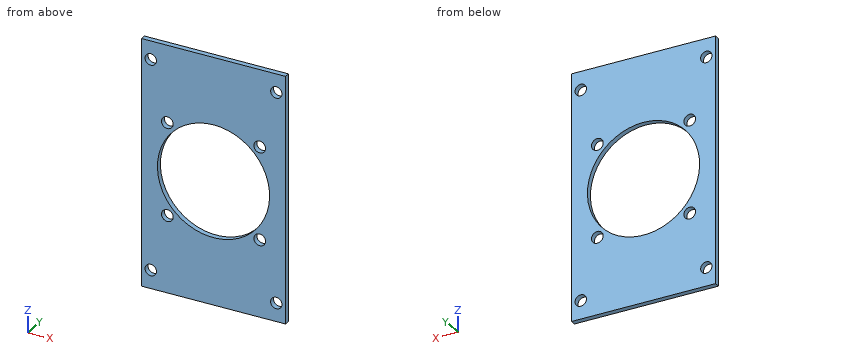
```python
from build123d import *

# Parameters (mm, degrees)
SKETCH1_W           = 86
SKETCH1_H           = 147
SKETCH1_R           = 33.5
SKETCH1_R_2         = 3.4
BOSS_EXTRUDE1_DEPTH = 3.175
SKETCH2_R           = 3.5
CUT_EXTRUDE1_DEPTH  = 10


with BuildPart() as part:
    # Sketch1 → Boss-Extrude1 (new body)
    with BuildSketch(Plane(origin=(0, 0, 0), x_dir=(1, 0, 0), z_dir=(0, 1, 0))):
        Rectangle(SKETCH1_W, SKETCH1_H)
        with Locations(Location((0, 0, 0), (0, 0, 270))):
            Circle(SKETCH1_R, mode=Mode.SUBTRACT)
        with Locations(Location((-37.5, -62.5, 0), (0, 0, 270))):
            Circle(SKETCH1_R_2, mode=Mode.SUBTRACT)
        with Locations(Location((37.5, -62.5, 0), (0, 0, 270))):
            Circle(SKETCH1_R_2, mode=Mode.SUBTRACT)
        with Locations(Location((-37.5, 62.5, 0), (0, 0, 270))):
            Circle(SKETCH1_R_2, mode=Mode.SUBTRACT)
        with Locations(Location((37.5, 62.5, 0), (0, 0, 270))):
            Circle(SKETCH1_R_2, mode=Mode.SUBTRACT)
    extrude(amount=BOSS_EXTRUDE1_DEPTH)

    # Sketch2 → Cut-Extrude1 (cut)
    with BuildSketch(Plane(origin=(0, 3.175, 0), x_dir=(1, 0, 0), z_dir=(0, 1, 0))):
        with Locations(Location((-27.577164466, 27.577164466, 0), (0, 0, 270))):
            Circle(SKETCH2_R)
        with Locations(Location((27.577164466, 27.577164466, 0), (0, 0, 270))):
            Circle(SKETCH2_R)
        with Locations(Location((27.577164466, -27.577164466, 0), (0, 0, 270))):
            Circle(SKETCH2_R)
        with Locations(Location((-27.577164466, -27.577164466, 0), (0, 0, 270))):
            Circle(SKETCH2_R)
    extrude(amount=-CUT_EXTRUDE1_DEPTH, mode=Mode.SUBTRACT)


solid = part.part
```
Input: part model. Units: mm. Frame: model coordinates. Round coordinates to 2 decimals unless told otherwise and drop trailing zeros. Order: outer loops, then holes, each group sorted by start corner. A loop starts at its lowest first (then second) coordinate and runs counter-clockwise, first axis right, second up. Notation, with made-up numbers: (16, 33) - (72, 33) arc R21 cw to (72, 51) - close; hole circle Ø11 at (69, 61.25). An arc over 180 degrees is marked (long way). Answer in a Markdown table with one row per item.
Item 1: Section query C-C (z = -62.5). Return the cut outline in (x, y) (3 decimals).
Model answer:
| item | result |
|---|---|
| outline | (-43, 0) - (-40.9, 0) - (-40.9, 3.175) - (-43, 3.175) - close; (-34.1, 0) - (34.1, 0) - (34.1, 3.175) - (-34.1, 3.175) - close; (40.9, 0) - (43, 0) - (43, 3.175) - (40.9, 3.175) - close |
Item 2: Section query D-D (x = -6). Return the cut outline in (y, z) (3 decimals).
Model answer:
| item | result |
|---|---|
| outline | (0, -73.5) - (3.175, -73.5) - (3.175, -32.958) - (0, -32.958) - close; (0, 32.958) - (3.175, 32.958) - (3.175, 73.5) - (0, 73.5) - close |
Item 3: Section query A-A (z = 0). Return the cut outline in (x, y) (3 decimals).
Model answer:
| item | result |
|---|---|
| outline | (-43, 0) - (-33.5, 0) - (-33.5, 3.175) - (-43, 3.175) - close; (33.5, 0) - (43, 0) - (43, 3.175) - (33.5, 3.175) - close |
Item 4: Pin query (flat end, axial travel): pin 1 (5.5 mm diameter, centred on x = 37.5, z = 62.5, fed in from -Y). Return the tip coordinate at first contact, or that it passes through.
Model answer:
| item | result |
|---|---|
| pin 1 | passes through |
Item 5: Line query: line 1 (Z direction, x = -30, y = 1.55); line 2 (X direction, y = 2.75, z = -25); line 3 (X direction, y = 1.8, z = -62.5). Output: solid intervals per line, ascending.
Model answer:
| item | result |
|---|---|
| line 1 | z = -73.5 to -30.1, -25.05 to -14.91, 14.91 to 25.05, 30.1 to 73.5 |
| line 2 | x = -43 to -29.95, -25.21 to -22.3, 22.3 to 25.21, 29.95 to 43 |
| line 3 | x = -43 to -40.9, -34.1 to 34.1, 40.9 to 43 |
Item 6: Section query B-B (x = 37.5). Return the cut outline in (y, z) (3 decimals).
Model answer:
| item | result |
|---|---|
| outline | (0, -73.5) - (3.175, -73.5) - (3.175, -65.9) - (0, -65.9) - close; (0, -59.1) - (3.175, -59.1) - (3.175, 59.1) - (0, 59.1) - close; (0, 65.9) - (3.175, 65.9) - (3.175, 73.5) - (0, 73.5) - close |
